Read the model definition and answer for the solid it produces. Units are mm, in the model's axes. A direction names the side the tool comes from. Round coordinates to 2 decimals unless told otherwise and drop trailing zeros. Order: outer loops, then holes, each group sorted by start corner. A loop starts at its lowest first (then second) coordinate and runs counter-clockwise, first axis right, second up. Notation, with made-up numbers: (38, 18) - (66, 18) arc R14 cw to (66, 38) - close; hole circle Ø5 at (-31.75, 39). An arc over 180 degrees is marked (long way). Answer as a JSON object with one key per item and string values. Group by question number.
Q1. A cutting plane is placed at C-C on x = 8.25. Determine the outline of the cut face in (y, z) (3 decimals), and give its area (3 significant figures).
Q2. A cutting plane is placed at A-A on z = 38.1. Determine the outline of the cut face in (x, y) (1 decimal).
Q3. A cutting plane is placed at D-D on z = 183. Determine the outline of the cut face in (x, y) (3 decimals).
Q4. The mould has two halves that part along Z. Classify faces 1 (the flat face through (13, -50.8, 146)), 2 (the flat face through (2, -27, 296.258)), 3 (the cylindrical face through (23.83, -13.35, 30.42)): pulls with the +Z half, pulls with the -Z half, needs draft (parallel to the pull), parting line crosses it, or undercut.
Q5. Consider line 1 (X direction, y = -3.5, z = 106.5) (3 decimals); line 2 (Y direction, x = 11, z = 218) (3 decimals); line 3 (Z direction, x = 2, y = -28). Determine where each line is inside the solid, lowest interval first.
Q6. A tool of negligible diameter and unlimited length cuts with its end or side. For faces 4 (the flat face through (0, -9, 146)), 5 (the flat face through (22.225, -41, 146)), from which of +Z, -Z, +X, -X, +Y, -Y can it reach the whole face along a straight path? Write none if from no direction.
Q7. A cutting plane is placed at B-B on y = -25.4. Count the separate pieces of the cut face and the enclosed holes in it, and give its area (3 significant figures).
Autodesk Inventor part; units mm, degrees
ref_plane "YZ Plane" through (0, 0, 0) normal (1, 0, 0) x (0, 1, 0)
ref_plane "XZ Plane" through (0, 0, 0) normal (0, 1, 0) x (-1, 0, 0)
ref_plane "XY Plane" through (0, 0, 0) normal (0, 0, 1) x (1, 0, 0)
sketch "Sketch1" plane through (0, 0, 0) normal (0, 0, 1) x (1, 0, 0)
  line L0 (0, 0) -> (25.4, 0)
  line L1 (25.4, 0) -> (25.4, -50.8)
  line L2 (25.4, -50.8) -> (0, -50.8)
  line L3 (0, -50.8) -> (0, 0)
  line L4 (22.225, -3.175) -> (3.175, -3.175)
  line L5 (3.175, -3.175) -> (3.175, -47.625)
  line L6 (3.175, -47.625) -> (22.225, -47.625)
  line L7 (22.225, -47.625) -> (22.225, -3.175)
  dimension "d0" = 25.4
  dimension "d1" = 50.8
  dimension "d2" = 3.175
extrude "Extrusion1" add sketch "Sketch1" along normal blind 296.258
sketch "Sketch2" plane through (25.4, -50.8, 0) normal (1, 0, 0) x (0, 0, -1)
  circle A0 centre (-38.1, 25.4) radius 14.2875
  circle A1 centre (-148.1252, 25.4) radius 14.2875
  line L0 (0, 50.8) -> (0, 0)
  line L1 (-296.258, 0) -> (-296.258, 50.8)
  line L2 (0, 0) -> (-296.258, 0)
  dimension "d5" = 38.1
  dimension "d6" = 110.0252
  dimension "d7" = 148.1328
  dimension "d8" = 25.4
  dimension "d9" = 25.4
  dimension "d10" = 28.575
  dimension "d11" = 28.575
extrude "Extrusion2" cut sketch "Sketch2" against normal blind 190.5
sketch "Sketch3" plane through (25.4, -50.8, 0) normal (1, 0, 0) x (0, 0, -1)
  circle A0 centre (-258.158, 25.4) radius 14.2875
  line L0 (-296.258, 0) -> (-296.258, 50.8)
  line L1 (0, 50.8) -> (-296.258, 50.8)
  circle A1 centre (-148.1252, 25.4) radius 14.2875
  dimension "d14" = 38.1
  dimension "d15" = 28.575
  dimension "d16" = 25.4
  dimension "d19" = 110.0328
extrude "Extrusion3" cut sketch "Sketch3" against normal blind 25.4 contours A0
properties part number "DRL SS"
Result set:
{
 "1": {"outline": "(-50.8, 0) - (-47.625, 0) - (-47.625, 296.258) - (-50.8, 296.258) - close; (-3.175, 0) - (0, 0) - (0, 296.258) - (-3.175, 296.258) - close", "area": "1,880 mm²"},
 "2": {"outline": "(0, -50.8) - (25.4, -50.8) - (25.4, -39.7) - (22.2, -39.7) - (22.2, -47.6) - (3.2, -47.6) - (3.2, -39.7) - (0, -39.7) - close; (0, -11.1) - (3.2, -11.1) - (3.2, -3.2) - (22.2, -3.2) - (22.2, -11.1) - (25.4, -11.1) - (25.4, 0) - (0, 0) - close"},
 "3": {"outline": "(0, -50.8) - (25.4, -50.8) - (25.4, 0) - (0, 0) - close; hole (3.175, -47.625) - (22.225, -47.625) - (22.225, -3.175) - (3.175, -3.175) - close"},
 "4": {"face 1": "needs draft", "face 2": "pulls with the +Z half", "face 3": "undercut"},
 "5": {"line 1": "x = 0 to 3.175, 22.225 to 25.4", "line 2": "y = -50.8 to -47.625, -3.175 to 0", "line 3": "z = 0 to 24.05, 52.15 to 134.08, 162.17 to 244.11, 272.21 to 296.26"},
 "6": {"face 4": "+Z, -Z, -X, +Y, -Y", "face 5": "+Z, -Z"},
 "7": {"separate pieces": "8", "enclosed holes": "0", "area": "1,340 mm²"}
}
